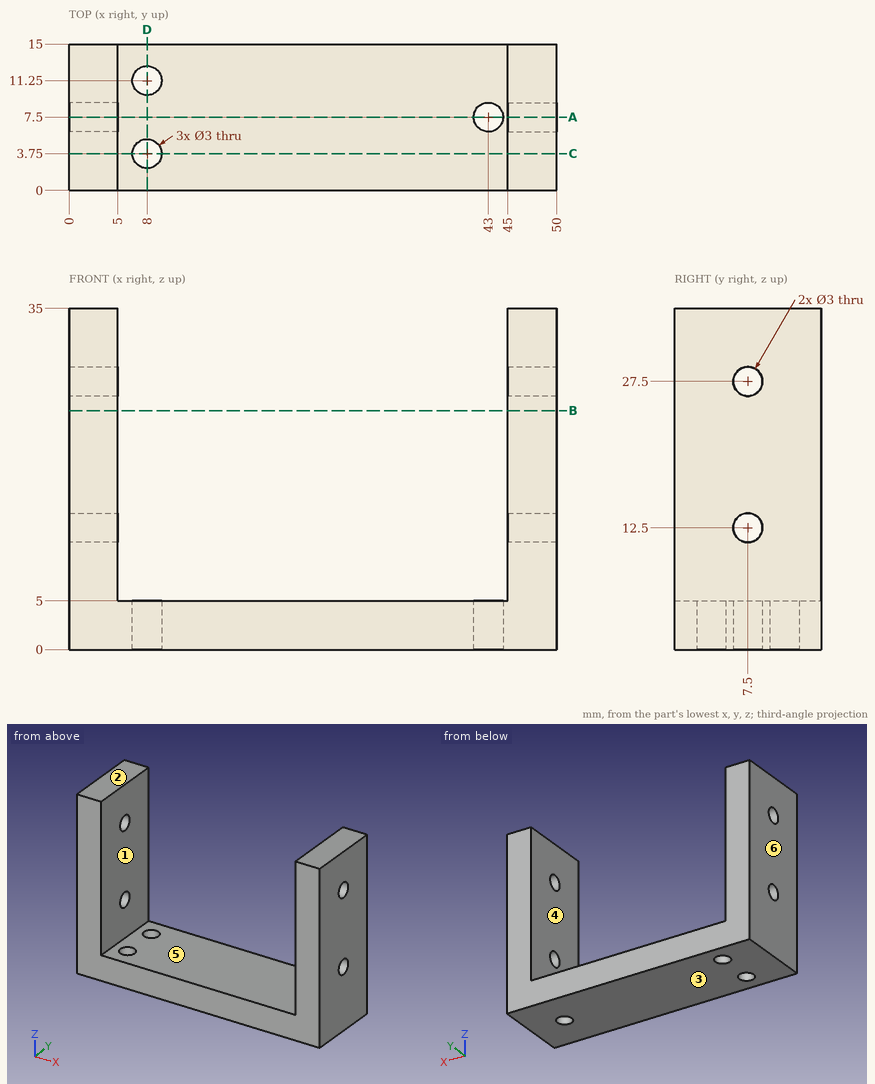
For this review, use the dimensioned drawing (mm, ordinates from the lowest corner) and the shaded views. A direction names the side the tool comes from. Round coordinates to 2 decimals unless told otherwise and drop trailing zeros. Order: outer loops, then holes, each group sorted by start corner. A loop starts at its lowest first (then second) coordinate and runs counter-clockwise, first axis right, second up. Notation, with made-up numbers: (9, -29) -> (46, -29) arc R32 ccw to (46, 9) -> close; hole circle Ø5 at (-35, 63.5). An arc over 180 degrees is marked (long way). Use CSV: the item, a comma, the result in double quotes. Start each with the question number.
(1) Mouldability with a two-part tool opening along X and no side actions: class the marked faces 3, 4, 5 and 6 as pulls with the +X half, pulls with the -X half, needs draft (parallel to the pull), parting line crosses it, or undercut.
(2) Consider section A-A on y = 7.5. Write out the cut boundary in (x, z), and give its area (3 significant figures).
(3) Consider section C-C on y = 3.75. Write out the cut boundary in (x, z).
(4) Consider section D-D on x = 8. Write out the cut boundary in (y, z).
(5) Tool access review of the marked faces 1 and 2: name each direction out of +Z, -Z, +X, -X, +Y, -Y from which nothing blocks a thin tool from reaching the whole face with its end or side.
(6) Consider section B-B on z = 24.5. Write out the cut boundary in (x, y).
(7) Wall thickness on probe 1 along X at (y, z) = (1.25, 16.5); probe 2 along Y at (x, z) = (47.25, 12.5); probe 3 along Z at (x, y) = (4, 8.5): over which ranges is each line inside the solid? List them lowest first. Write a range as from..to.
(8) Insertion check: pin 1 (5 mm diameter, centred on x = 8, y = 11.25, fed in from +Z). The pin has a flat end and moves straight along its axis. Give the tip position at first contact, or say it passes through.
Responses:
1,face 3,"needs draft"
1,face 4,"undercut"
1,face 5,"undercut"
1,face 6,"pulls with the -X half"
2,outline,"(0, 0) -> (41.5, 0) -> (41.5, 5) -> (5, 5) -> (5, 11) -> (0, 11) -> close; (0, 14) -> (5, 14) -> (5, 26) -> (0, 26) -> close; (0, 29) -> (5, 29) -> (5, 35) -> (0, 35) -> close; (44.5, 0) -> (50, 0) -> (50, 11) -> (45, 11) -> (45, 5) -> (44.5, 5) -> close; (45, 14) -> (50, 14) -> (50, 26) -> (45, 26) -> close; (45, 29) -> (50, 29) -> (50, 35) -> (45, 35) -> close"
2,area,"475 mm²"
3,outline,"(0, 0) -> (6.5, 0) -> (6.5, 5) -> (5, 5) -> (5, 35) -> (0, 35) -> close; (9.5, 0) -> (50, 0) -> (50, 35) -> (45, 35) -> (45, 5) -> (9.5, 5) -> close"
4,outline,"(0, 0) -> (2.25, 0) -> (2.25, 5) -> (0, 5) -> close; (5.25, 0) -> (9.75, 0) -> (9.75, 5) -> (5.25, 5) -> close; (12.75, 0) -> (15, 0) -> (15, 5) -> (12.75, 5) -> close"
5,face 1,"+Z, +Y, -Y"
5,face 2,"+Z, +X, -X, +Y, -Y"
6,outline,"(0, 0) -> (5, 0) -> (5, 15) -> (0, 15) -> close; (45, 0) -> (50, 0) -> (50, 15) -> (45, 15) -> close"
7,probe 1,"0..5, 45..50"
7,probe 2,"0..6, 9..15"
7,probe 3,"0..11.38, 13.62..26.38, 28.62..35"
8,pin 1,"z = 5"
